Geometry check sheet. Reference: the model listing, model coordinates, mm. Face numbers are marked on the shaded views. Round coordinates to 2 decimals unless told otherwise and drop trailing zeros. Order: outer loops, then holes, each group sorted by start corner. A loop starts at its lowest first (then second) coordinate and runs counter-clockwise, first axis right, second up.
(1) Go/stop test with flat-tipped pins: pin 1 (5.5 mm diameter, centred on x = -19.05, z = -7.94, fed in from +Y); pin 2 (3.5 mm diameter, centred on x = 19.05, z = -7.94, fed in from -Y); pin 3 (6 mm diameter, centred on x = -16.5, z = -5.5, fed in from +Y). Record where each tip stops, or that it passes through.
(2) Sectioned sample at A-A (x = 0). Record the boundary of the cut face in (y, z).
(3) Material ranges on line 1 along Z through (x, y) = (-19, -41); line 2 along Y through (x, z) = (0, -5); line 3 along Y through (x, z) = (-9, -9.25), recorded low to high.
(4) Release check for a two-part mould opening along Y. For the marked faces 1, 2 and 3 record: +Y half, -Y half, draft (parallel to the pull), parting line (faces both ways), or undercut.
(5) Sectioned sample at C-C (z = -3.5). Record the boundary of the cut face in (x, y).
(6) Sectioned sample at D-D (y = 36.5). Record the boundary of the cut face in (x, z), plus the area to 3 significant figures.
(7) Sectioned sample at B-B (y = 0). Record the boundary of the cut face in (x, z).
from build123d import *

# Parameters (mm, degrees)
SKETCH1_R                  = 25.4
BOSS_EXTRUDE1_DEPTH        = 12.7
F_10_32_TAPPED_HOLE1_D     = 4.0386
F_10_32_TAPPED_HOLE1_DEPTH = 12.02944
F_10_32_TAPPED_HOLE1_TIP   = 1.213317848


with BuildPart() as part:
    # Sketch1 → Boss-Extrude1 (new body, symmetric)
    with BuildSketch(Plane.XY):
        with BuildLine():
            Line((38.1, -44.45), (-38.1, -44.45))
            Line((-38.1, -44.45), (-38.1, 19.05))
            ThreePointArc((-38.1, 19.05), (-30.660512242, 37.010512242), (-12.7, 44.45))
            Line((-12.7, 44.45), (12.7, 44.45))
            ThreePointArc((12.7, 44.45), (30.660512242, 37.010512242), (38.1, 19.05))
            Line((38.1, 19.05), (38.1, -44.45))
        make_face()
        Circle(SKETCH1_R, mode=Mode.SUBTRACT)
    extrude(amount=BOSS_EXTRUDE1_DEPTH, both=True)

    # #10-32 Tapped Hole1
    with Locations(Plane(origin=(0, -44.45, 0), x_dir=(-1, 0, 0), z_dir=(0, -1, 0))):
        with Locations((19.05, -7.9375), (-19.05, -7.9375), (-19.05, 7.9375), (19.05, 7.9375)):
            Hole(F_10_32_TAPPED_HOLE1_D / 2, depth=F_10_32_TAPPED_HOLE1_DEPTH)
            with Locations((0, 0, -(F_10_32_TAPPED_HOLE1_DEPTH + F_10_32_TAPPED_HOLE1_TIP / 2))):  # 118° drill point
                Cone(0, F_10_32_TAPPED_HOLE1_D / 2, F_10_32_TAPPED_HOLE1_TIP, mode=Mode.SUBTRACT)


solid = part.part
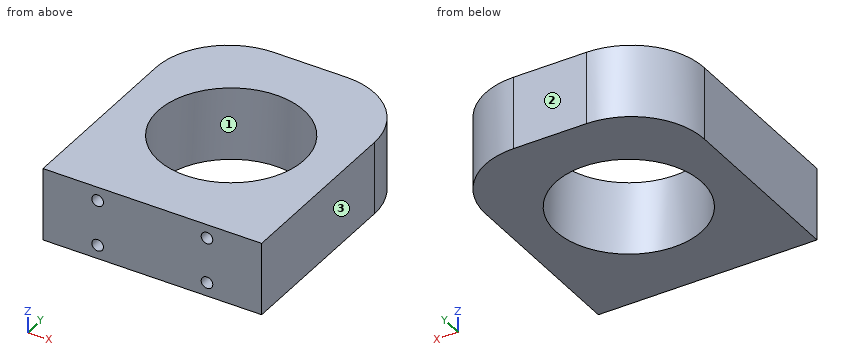
Answer below:
1. pin 1: stops at y = 44.19
1. pin 2: stops at y = -32.26
1. pin 3: stops at y = 44.44
2. outline: (-44.45, -12.7) - (-25.4, -12.7) - (-25.4, 12.7) - (-44.45, 12.7) - close; (25.4, -12.7) - (44.45, -12.7) - (44.45, 12.7) - (25.4, 12.7) - close
3. line 1: z = -12.7 to -9.96, -5.92 to 5.92, 9.96 to 12.7
3. line 2: y = -44.45 to -25.4, 25.4 to 44.45
3. line 3: y = -44.45 to -23.75, 23.75 to 44.45
4. face 1: undercut
4. face 2: +Y half
4. face 3: draft
5. outline: (-38.1, -44.45) - (38.1, -44.45) - (38.1, 19.05) arc R25.4 ccw to (12.7, 44.45) - (-12.7, 44.45) arc R25.4 ccw to (-38.1, 19.05) - close; hole circle Ø50.8 at (0, 0)
6. outline: (-31.16, -12.7) - (31.16, -12.7) - (31.16, 12.7) - (-31.16, 12.7) - close
6. area: 1,580 mm2
7. outline: (-38.1, -12.7) - (-25.4, -12.7) - (-25.4, 12.7) - (-38.1, 12.7) - close; (25.4, -12.7) - (38.1, -12.7) - (38.1, 12.7) - (25.4, 12.7) - close
